Build history of the part. All positions in model axes, mm. A direction names the side the tool comes from. Give positions to 0.01 mm unless a question says otherwise; leave off trailing zeros. Loops run counter-clockwise (first coordinate to the right, second up) from the corner with the lowest first, then second, coordinate; pieces in that order, holes last. Notation, with made-up numbers: (-4, 35.5) -> (41, 35.5) arc R37 cw to (41, 74.5) -> close; hole circle Ø3 at (-32.5, 5). An arc over 180 degrees is marked (long way). One line per question, with ' | ' between items. Start each with the question number.
(1) Mould opens along X. For faces 4 (the face through (88, -1, 2)), 5 (the face through (82, 47.5, 0.7)), 6 (the face through (-65, -1, 10)) say: pulls with the +X half, pulls with the -X half, needs draft (parallel to the pull), parting line crosses it, or undercut.
(2) Drill centre lines: L1, parallel to X at y = -46, z = 4.1; L2, parallel to Y at x = 78, z = 3.25; L3, parallel to Z at x = -27, y = -38. Where is each one in solid material? Low to high. Write a range as from..to.
(3) Slice it at A-A, the plane y = -35.5. Write the cut outline in (x, z).
(4) 3-axis set-ups, long thin cutter, end or side, ignore diameter. For faces 1 (the face through (-84, -44, 1.5)), 2 (the face through (6.3, -1.3, 10)), 3 (the face through (-59.185, 1.201, 7.465)): which of +Z, -Z, +X, -X, +Y, -Y reach the whole face in a straight line?
(5) Flat gauge pins, fed straight in: pin 1 Ø5 at (x, z) = (-12, 6) entering from +Y; pin 2 Ø1 at (x, y) = (55, 3) entering from +Z; pin 3 Ø2.5 at (x, y) = (83.5, 47) entering from -Z. Where does each tip first touch, or does it go through?
(6) Slice it at B-B, the plane x = -49. Write the cut outline in (y, z), then the cut area to 3 significant figures.
```python
from build123d import *

# Parameters (mm, degrees)
F0_W     = 176
F0_H     = 100
F0_R     = 4
F0_R_2   = 3
F1_DEPTH = 5
F0_R_3   = 2
F0_R_4   = 1.5
F2_DEPTH = 10
F4_R     = 1.5
F5_DEPTH = 10.001
F4_R_2   = 2.5
F6_DEPTH = 1.5


with BuildPart() as f1:
    # F0 (on Top) → F1 (new body)
    with BuildSketch(Plane.XY):
        Rectangle(F0_W, F0_H)
        with Locations((-63, 0)):
            Circle(F0_R, mode=Mode.SUBTRACT)
        with Locations((-15, 0)):
            Circle(F0_R, mode=Mode.SUBTRACT)
        with Locations((5, 0)):
            Circle(F0_R_2, mode=Mode.SUBTRACT)
        with Locations((78, 0)):
            Circle(F0_R_2, mode=Mode.SUBTRACT)
    extrude(amount=F1_DEPTH)

    # F0 (on Top) → F2 (join)
    with BuildSketch(Plane.XY):
        with Locations((-63, 0)):
            Circle(F0_R)
        with Locations((-63, 0)):
            Circle(F0_R_3, mode=Mode.SUBTRACT)
        with Locations((-15, 0)):
            Circle(F0_R)
        with Locations((-15, 0)):
            Circle(F0_R_3, mode=Mode.SUBTRACT)
        with Locations((5, 0)):
            Circle(F0_R_2)
        with Locations((5, 0)):
            Circle(F0_R_4, mode=Mode.SUBTRACT)
        with Locations((78, 0)):
            Circle(F0_R_2)
        with Locations((78, 0)):
            Circle(F0_R_4, mode=Mode.SUBTRACT)
    extrude(amount=F2_DEPTH)

    # F4 (on face) → F5 (cut, through all)
    with BuildSketch(Plane(origin=(0, 0, 0), x_dir=(1, 0, 0), z_dir=(0, 0, -1))):
        with Locations((-84, 46)):
            Circle(F4_R)
        with Locations((-84, -46)):
            Circle(F4_R)
        with Locations((84, 46)):
            Circle(F4_R)
        with Locations((84, -46)):
            Circle(F4_R)
    extrude(amount=-F5_DEPTH, mode=Mode.SUBTRACT)

    # F4 (on face) → F6 (cut)
    with BuildSketch(Plane(origin=(0, 0, 0), x_dir=(1, 0, 0), z_dir=(0, 0, -1))):
        with Locations((84, -46)):
            Circle(F4_R_2)
        with Locations((84, -46)):
            Circle(F4_R, mode=Mode.SUBTRACT)
        with Locations((84, 46)):
            Circle(F4_R_2)
        with Locations((84, 46)):
            Circle(F4_R, mode=Mode.SUBTRACT)
        with Locations((-84, 46)):
            Circle(F4_R_2)
        with Locations((-84, 46)):
            Circle(F4_R, mode=Mode.SUBTRACT)
        with Locations((-84, -46)):
            Circle(F4_R_2)
        with Locations((-84, -46)):
            Circle(F4_R, mode=Mode.SUBTRACT)
    extrude(amount=-F6_DEPTH, mode=Mode.SUBTRACT)


solid = f1.part
```
Final values:
1) face 4: pulls with the +X half | face 5: undercut | face 6: needs draft
2) L1: -88..-85.5, -82.5..82.5, 85.5..88 | L2: -50..-1.5, 1.5..50 | L3: 0..5
3) outline: (-88, 0) -> (88, 0) -> (88, 5) -> (-88, 5) -> close
4) face 1: -Z | face 2: +Z, +X, -X, +Y, -Y | face 3: +Z
5) pin 1: y = 50 | pin 2: z = 5 | pin 3: z = 1.5
6) outline: (-50, 0) -> (50, 0) -> (50, 5) -> (-50, 5) -> close | area: 500 mm2
